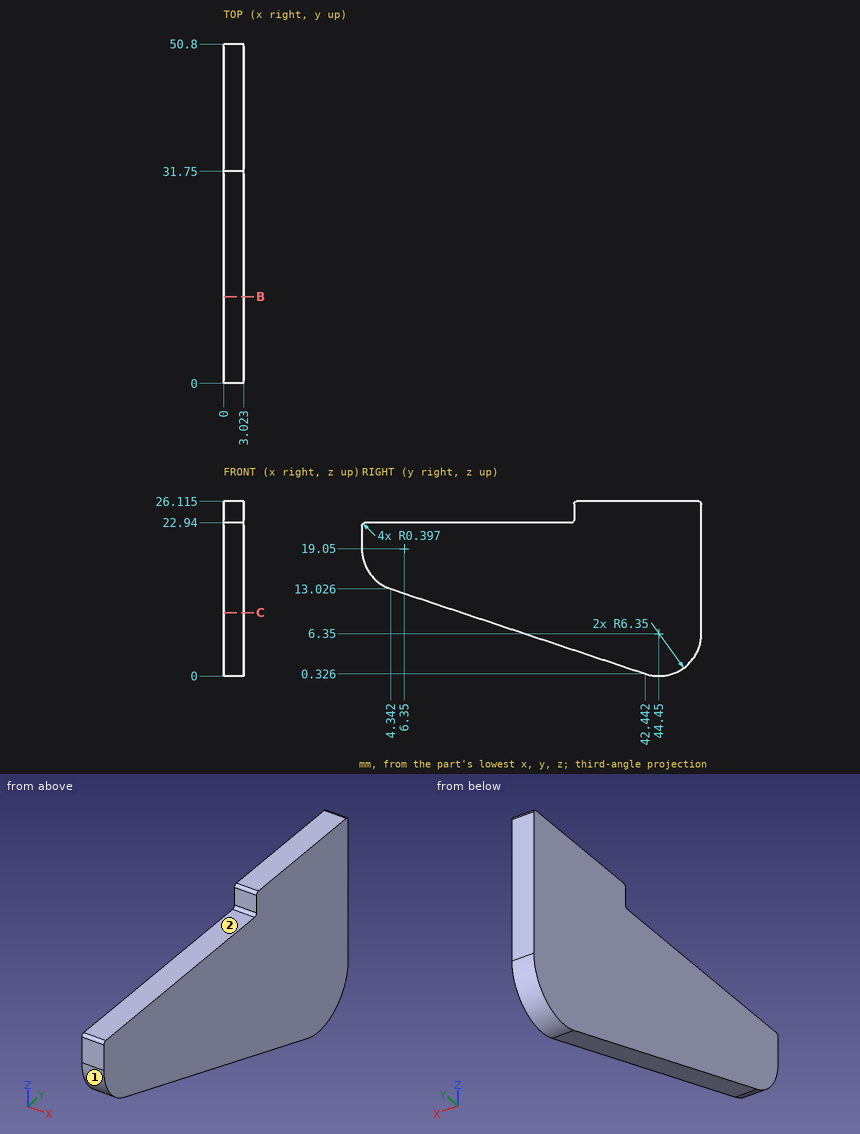
Answer from the drawing. Dimensions are ordinates in mm from the lowest x, y and z of the part. A direction names the side the tool comes from. Give positions to 0.01 mm unless a question says otherwise; leave off trailing zeros. Order: outer loops, then holes, each group sorted by start corner. A loop starts at its lowest first (then second) coordinate and runs counter-clockwise, first axis right, second up. Notation, with made-up numbers: (46, -38.75) -> (93, -38.75) arc R35 ccw to (93, -4.75) -> close; hole circle Ø4 at (-30, -18). An arc over 180 degrees is marked (long way). One line per item, written item: value.
Item 1: Straight lines are drawn through the part: probe 1 along Z at (x, y) = (0.1, 23.5); probe 2 along Z at (x, y) = (2.3, 35) (1 decimal). For each, find the intervals that lie inside material, in ascending order.
Answer sheet:
probe 1: 6.64 to 22.94
probe 2: 2.8 to 26.1
Item 2: Find section C-C, the plane z = 9.5. Give the vertices of the cut face in (x, y).
Answer sheet:
outline: (0, 14.92) -> (3.02, 14.92) -> (3.02, 50.8) -> (0, 50.8) -> close
Item 3: A tool of negligible diameter and unlimited length cuts with its end or side. For the marked faces 1 and 2, from which of +Z, -Z, +X, -X, +Y, -Y can it reach the whole face along a straight path? Write none if from no direction.
Answer sheet:
face 1: -Z, +X, -X, -Y
face 2: +Z, +X, -X, -Y
Item 4: Find section B-B, the plane y = 13. Give the vertices of the cut face in (x, z).
Answer sheet:
outline: (0, 10.14) -> (3.02, 10.14) -> (3.02, 22.94) -> (0, 22.94) -> close
